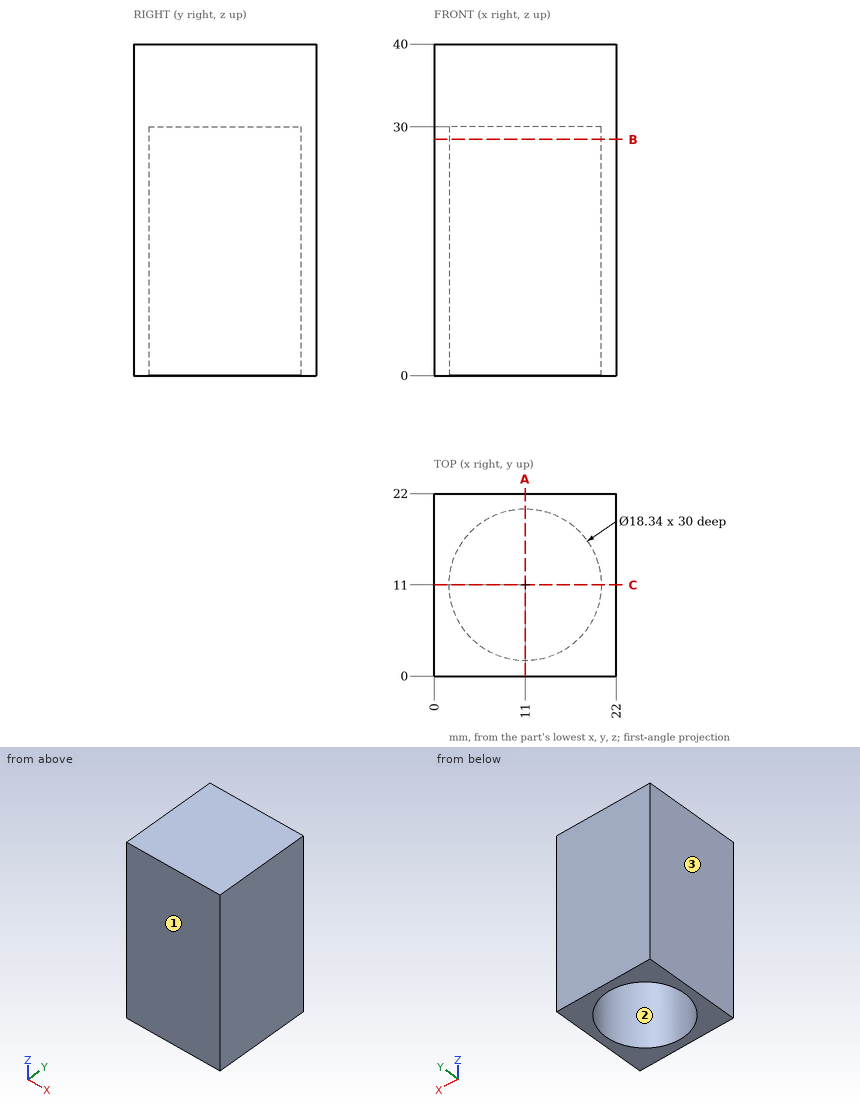
The drawing under review shows one solid part. Ordinate dimensions are in mm from its lowest x, y, z. Coordinates: 2 decimals unless noted, no trailing zeros. Loops run counter-clockwise (first coordinate to the right, second up) from the corner with the lowest first, then second, coordinate; pieces in that order, holes last. Notation, with made-up numbers: (26.25, 81) - (42.25, 81) arc R29 ccw to (42.25, 120) - close; hole circle Ø9 at (16, 68). An arc over 180 degrees is marked (long way). Return JSON: item names as keys, results as strings.
Item 1: For line 1 (Y direction, x = 11, z = 16.5); line 2 (Z direction, x = 8.5, y = 8.5), list the stretches that pass through material, from the lowest coordinate up.
Determined:
{"line 1": "y = 0 to 1.83, 20.17 to 22", "line 2": "z = 30 to 40"}
Item 2: Insertion check: pin 1 (9 mm diameter, centred on x = 14, y = 7, fed in from -Z). The pin has a flat end and moves straight along its axis. Give the tip position at first contact, or say it passes through.
Determined:
{"pin 1": "stops at z = 0"}
Item 3: Take a section at B-B (z = 28.5). Give the boundary of the cut face in (x, y), then the cut area to 3 significant figures.
Determined:
{"outline": "(0, 0) - (22, 0) - (22, 22) - (0, 22) - close; hole circle Ø18.34 at (11, 11)", "area": "220 mm2"}
Item 4: Take a section at A-A (x = 11). Give the boundary of the cut face in (y, z).
Determined:
{"outline": "(0, 0) - (1.83, 0) - (1.83, 30) - (20.17, 30) - (20.17, 0) - (22, 0) - (22, 40) - (0, 40) - close"}
Item 5: Mouldability with a two-part tool opening along X and no side actions: class the marked faces 1, 2 and 3 as pulls with the +X half, pulls with the -X half, needs draft (parallel to the pull), parting line crosses it, or undercut.
Determined:
{"face 1": "needs draft", "face 2": "undercut", "face 3": "pulls with the -X half"}
